Geometry: final body of the model. Coordinates: model frame, mm. A direction names the side the tool comes from. Give positions to 0.01 mm unless a question says otherwise; leave off trailing zeros. Order: outer loops, then holes, each group sorted by start corner. A loop starts at its lowest first (then second) coordinate and runs counter-clockwise, first axis right, second up. Notation, with made-up numbers: (-27.5, -19) - (-16.5, -19) arc R26 ccw to (-16.5, 1) - close; hole circle Ø1 at (32.5, 24.5). An arc over 180 degrees is marked (long way). One line per item, written item: value.
```python
from build123d import *

# Parameters (mm, degrees)
BOSS_EXTRUDE1_DEPTH = 2
SKETCH2_R           = 9
CUT_EXTRUDE1_DEPTH  = 3
FILLET1_R           = 4
SKETCH4_R           = 1.5
CUT_EXTRUDE2_DEPTH  = 3.0000001
CUT_EXTRUDE3_DEPTH  = 3.0000001


with BuildPart() as part:
    # Sketch1 → Boss-Extrude1 (new body)
    with BuildSketch(Plane(origin=(0, 0, 0), x_dir=(1, 0, 0), z_dir=(0, 1, 0))):
        with BuildLine():
            Line((0, 27.5), (0, 17.5))
            ThreePointArc((0, 17.5), (13.287682266, 12.507351161), (20, 0))
            ThreePointArc((20, 0), (14.277242376, -15.051993223), (0, -22.5))
            ThreePointArc((0, -22.5), (-17.510327053, -16.817030059), (-25, 0))
            ThreePointArc((-25, 0), (-17.815844528, 18.582585934), (0, 27.5))
        make_face()
    extrude(amount=BOSS_EXTRUDE1_DEPTH)

    # Sketch2 → Cut-Extrude1 (cut, through all)
    with BuildSketch(Plane(origin=(0, 2, 0), x_dir=(1, 0, 0), z_dir=(0, 1, 0))):
        Circle(SKETCH2_R)
    extrude(amount=-CUT_EXTRUDE1_DEPTH, mode=Mode.SUBTRACT)

    # Fillet1
    fillet1_edges = [part.edges().sort_by_distance(p)[0] for p in [
        (0, 1, -27.5),
        (0, 1, -17.5),
        (20, 1, 0),
        (0, 1, 22.5),
    ]]
    fillet(fillet1_edges, radius=FILLET1_R)

    # Sketch4 → Cut-Extrude2 (cut, through all)
    with BuildSketch(Plane(origin=(0, 2, 0), x_dir=(1, 0, 0), z_dir=(0, 1, 0))):
        with Locations((-5.773502692, 10)):
            Circle(SKETCH4_R)
        with Locations((11.547005384, 0)):
            Circle(SKETCH4_R)
        with Locations((-5.773502692, -10)):
            Circle(SKETCH4_R)
    extrude(amount=-CUT_EXTRUDE2_DEPTH, mode=Mode.SUBTRACT)

    # Sketch5 → Cut-Extrude3 (cut, through all)
    with BuildSketch(Plane(origin=(0, 2, 0), x_dir=(1, 0, 0), z_dir=(0, 1, 0))):
        with BuildLine():
            ThreePointArc((-18.651783434, -4.132756796), (-17.097956543, -8.522240669), (-14.528379596, -12.405437933))
            ThreePointArc((-14.528379596, -12.405437933), (-11.787650951, -12.621464013), (-11.571624871, -9.880735369))
            ThreePointArc((-11.571624871, -9.880735369), (-13.618252323, -6.787830084), (-14.855850898, -3.291675511))
            ThreePointArc((-14.855850898, -3.291675511), (-17.174357809, -1.814249886), (-18.651783434, -4.132756796))
        make_face()
        with BuildLine():
            ThreePointArc((-1.191040224, -16.957696658), (6.508856337, -15.704039033), (12.837977748, -11.143086651))
            ThreePointArc((12.837977748, -11.143086651), (12.664068084, -8.682433661), (10.203415094, -8.856343325))
            ThreePointArc((10.203415094, -8.856343325), (5.173132739, -12.481313807), (-0.946619322, -13.477700417))
            ThreePointArc((-0.946619322, -13.477700417), (-2.808827894, -15.095488087), (-1.191040224, -16.957696658))
        make_face()
        with BuildLine():
            ThreePointArc((-8.627267861, 17.525882988), (-14.425164825, 13.171975745), (-18.235670183, 7.003331939))
            ThreePointArc((-18.235670183, 7.003331939), (-17.195996196, 4.667190222), (-14.859854479, 5.706864208))
            ThreePointArc((-14.859854479, 5.706864208), (-11.754755816, 10.733559053), (-7.03017458, 14.281464197))
            ThreePointArc((-7.03017458, 14.281464197), (-6.206511825, 16.702220233), (-8.627267861, 17.525882988))
        make_face()
    extrude(amount=-CUT_EXTRUDE3_DEPTH, mode=Mode.SUBTRACT)


solid = part.part
```
1) First-contact query: pin 1 (1 mm diameter, centred on y = 0.5, z = -7, fed in from -X); pin 2 (1 mm diameter, centred on x = -15, y = 1, fed in from +Z). Flat tips, straight axial feed; report the tip coordinate or a pass-through.
Answers below:
pin 1: x = -24.22
pin 2: z = 19.1
2) Section B-B, the plane z = -15. Return loops of the section in (x, y), then the cut area to 3 significant figures.
Answers below:
outline: (-20.57, 0) - (-12.51, 0) - (-12.51, 2) - (-20.57, 2) - close; (-6.26, 0) - (9.73, 0) - (9.73, 2) - (-6.26, 2) - close
area: 48.1 mm^2
3) Mould query, pull axis Z, two halves, no side actions, for faces 1 (the face through (0, 1, -22)), 2 (the face through (-17.312, 0.986, 16.993)), 3 (the face through (-17.1, 1, 1.8)), 4 (the face through (5.25, 1.01, 12.45)). Classes: released by +Z, released by -Z, zero draft, split by the parting line, or undercut.
Answers below:
face 1: zero draft
face 2: released by +Z
face 3: undercut
face 4: undercut
4) Section C-C, the plane z = -10. Return loops of the section in (x, y).
Answers below:
outline: (-23.13, 0) - (-16.78, 0) - (-16.78, 2) - (-23.13, 2) - close; (-12.38, 0) - (-7.27, 0) - (-7.27, 2) - (-12.38, 2) - close; (-4.27, 0) - (15.7, 0) - (15.7, 2) - (-4.27, 2) - close
5) Material intervals for line 1 along X through (y, z) = (0.95, 0); line 2 along Z through (x, y) = (8, 1.65); line 3 along Z through (x, y) = (-13, 1.65), sorted ascending.
Answers below:
line 1: -25 to -9, 9 to 10.05, 13.05 to 19.99
line 2: -15.85 to -4.12, 4.12 to 10.89, 15 to 19.99
line 3: -22.78 to -14.58, -9.19 to 7.91, 13.09 to 19.97
6) Section D-D, the plane y = 0.85. Count the separate pieces of the cut face and the enclosed holes in it, then the cut area to 3 significant figures.
Answers below:
separate pieces: 1
enclosed holes: 7
area: 1,150 mm^2
7) Section A-A, the plane x = 2. Return loops of the section in (y, z).
Answers below:
outline: (0, -17.7) - (2, -17.7) - (2, -8.77) - (0, -8.77) - close; (0, 8.77) - (2, 8.77) - (2, 13.36) - (0, 13.36) - close; (0, 16.88) - (2, 16.88) - (2, 22.17) - (0, 22.17) - close
8) Set-up query: faces 5 (the face through (-7, 0, -8)), 6 (the face through (-2.806, 1.014, 15.057)). Return all of +Z, -Z, +X, -X, +Y, -Y with unobstructed straight access to the full face (end or side cutting, diameter ignored); none if empty.
Answers below:
face 5: +Z, -Z, +X, -X, -Y
face 6: +Y, -Y
